Autodesk Inventor part; units mm, degrees
ref_plane "YZ Plane" through (0, 0, 0) normal (1, 0, 0) x (0, 1, 0)
ref_plane "XZ Plane" through (0, 0, 0) normal (0, 1, 0) x (-1, 0, 0)
ref_plane "XY Plane" through (0, 0, 0) normal (0, 0, 1) x (1, 0, 0)
sketch "Sketch1" plane through (0, 0, 0) normal (0, 0, 1) x (1, 0, 0)
  line L0 (0, 0) -> (9.5, 0)
  line L1 (9.5, 0) -> (9.5, 9.5)
  line L2 (9.5, 9.5) -> (0, 9.5)
  line L3 (0, 9.5) -> (0, 0)
  dimension "d0" = 9.5
  dimension "d1" = 9.5
extrude "Extrusion1" add sketch "Sketch1" along normal blind 9
sketch "Sketch2" plane through (9.5, 0, 0) normal (1, 0, 0) x (0, 0, -1)
  circle A0 centre (-15.25, 4.75) radius 4.75 construction
  line L0 (0, 0) -> (0, 9.5)
  line L1 (-9, 0) -> (-9, 9.5)
  line L2 (-9, 9.5) -> (-15.25, 9.5)
  line L3 (-9, 0) -> (-15.25, 0)
  arc A1 (-15.25, 9.5) -> (-15.25, 0) centre (-15.25, 4.75) ccw
  circle A2 centre (-15.25, 4.75) radius 1.5
  point P0 (0, 4.75)
  point P1 (0, 4.75)
  dimension "d4" = 9.5
  dimension "d5" = 15.25
  dimension "d6" = 3
extrude "Extrusion2" add sketch "Sketch2" against normal blind 3
sketch "Sketch3" plane through (0, 0, 0) normal (-1, 0, 0) x (0, 0, 1)
  circle A0 centre (15.25, 4.75) radius 1.5
  line L0 (9, 0) -> (9, 9.5)
  line L1 (9, 0) -> (15.25, 0)
  arc A1 (15.25, 0) -> (15.25, 9.5) centre (15.25, 4.75) ccw
  line L2 (15.25, 9.5) -> (9, 9.5)
  point P0 (0, 0)
extrude "Extrusion3" add sketch "Sketch3" against normal blind 3
fillet "Fillet1" radius 2 6 edges at (0, 4.75, 20) (0, 0, 7.625) (0, 9.5, 7.625) (9.5, 4.75, 20) (9.5, 0, 7.625) (9.5, 9.5, 7.625)
sketch "Sketch4" plane through (0, 0, 0) normal (0, 0, -1) x (-1, 0, 0)
  circle A0 centre (-4.75, 4.75) radius 2
  line L0 (-7.5, 9.5) -> (-2, 9.5)
  line L1 (0, 7.5) -> (0, 2)
  point P0 (0, 0)
  point P1 (0, 4.75)
  point P2 (-4.75, 9.5)
  dimension "d12" = 4
extrude "Extrusion4" cut sketch "Sketch4" against normal through all
sketch "Sketch5" plane through (0, 0, 9) normal (0, 0, 1) x (1, 0, 0)
  circle A0 centre (4.75, 4.75) radius 2
  circle A1 centre (4.75, 4.75) radius 3
  point P0 (0, 0)
  dimension "d15" = 6
extrude "Extrusion5" cut sketch "Sketch5" along normal blind 15 and the other way blind 6
properties part number "Arm6" material "ABS Plastic"
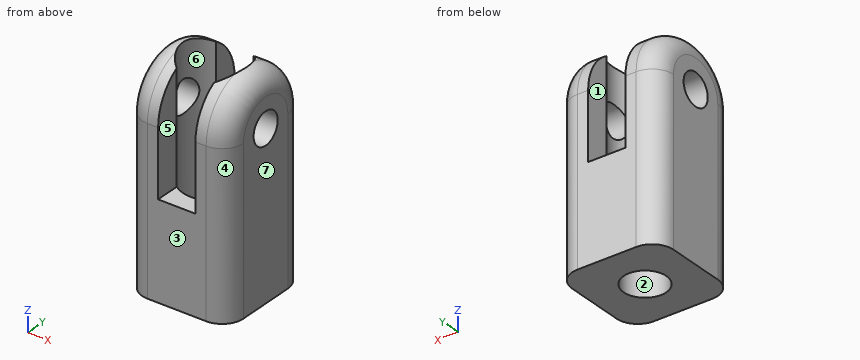
Here's how the part is built. I have some questions about the finished solid (model axes, mm). Face numbers are marked on the shaded views. A direction names the side the tool comes from. Round coordinates to 2 decimals unless told otherwise and drop trailing zeros. Write each loop counter-clockwise with the first axis right and the second up, starting at its lowest first coordinate (ties: lowest second). Pieces come first, ordered by that corner, then holes.
1. I need wall thicknesses on L1, parallel to X at y = 4.75, z = 13.25; L2, parallel to X at y = 2, z = 11; L3, parallel to Z at x = 6.25, y = 0.75. Which ranges of each line are inside material? Lowest first, please.
2. Suppose I cut it at C-C (z = 1.75). List the corners of the cut face in (x, y) for me, and give its area (4 significant figures).
3. If we mould it in two halves opening along X, with no side actions, what happens to the marked faces 1, 2, 3 and 4? For each: released by +X, released by -X, zero draft, split by the parting line, or undercut.
4. Suppose I cut it at B-B (x = 4.75). List the corners of the cut face in (y, z) for me, and give its area (3 significant figures).
5. For the marked faces 5, 6 and 7, which set-ups out of +Z, -Z, +X, -X, +Y, -Y let a thin tool reach every point of the face, with its end or its side?
6. Suppose I cut it at D-D (z = 11). List the corners of the cut face in (x, y) for me.
7. Suppose I cut it at A-A (y = 4.75). List the corners of the cut face in (x, z) for me.
8. Will these pins go through, and if not, where does the flat tip stop? pin 1 Ø1.2 at (x, y) = (4.5, 1) entering from +Z; pin 2 Ø1.2 at (y, z) = (0.5, 12.5) entering from +X; pin 3 Ø3 at (x, y) = (6, 4) entering from +Z.
Answer sheet:
1. L1: x = 0 to 1.75, 7.75 to 9.5
1. L2: x = 0 to 3, 6.5 to 9.5
1. L3: z = 0 to 9
2. outline: (0, 2) arc R2 ccw to (2, 0) - (7.5, 0) arc R2 ccw to (9.5, 2) - (9.5, 7.5) arc R2 ccw to (7.5, 9.5) - (2, 9.5) arc R2 ccw to (0, 7.5) - close; hole circle Ø4 at (4.75, 4.75)
2. area: 74.25 mm2
3. face 1: undercut
3. face 2: undercut
3. face 3: zero draft
3. face 4: released by +X
4. outline: (0, 0) - (2.75, 0) - (2.75, 3) - (1.75, 3) - (1.75, 9) - (0, 9) - close; (6.75, 0) - (9.5, 0) - (9.5, 9) - (7.75, 9) - (7.75, 3) - (6.75, 3) - close
4. area: 37.5 mm2
5. face 5: +Z, +Y, -Y
5. face 6: +Z
5. face 7: +Z, -Z, +X, +Y, -Y
6. outline: (0, 2) arc R2 ccw to (2, 0) - (3, 0) - (3, 2.31) arc R3 cw to (3, 7.19) - (3, 9.5) - (2, 9.5) arc R2 ccw to (0, 7.5) - close; (6.5, 0) - (7.5, 0) arc R2 ccw to (9.5, 2) - (9.5, 7.5) arc R2 ccw to (7.5, 9.5) - (6.5, 9.5) - (6.5, 7.19) arc R3 cw to (6.5, 2.31) - close
7. outline: (0, 0) - (2.75, 0) - (2.75, 3) - (1.75, 3) - (1.75, 13.75) - (0, 13.75) - close; (0, 16.75) - (1.75, 16.75) - (1.75, 19.98) arc R2 ccw to (0, 18) - close; (6.75, 0) - (9.5, 0) - (9.5, 13.75) - (7.75, 13.75) - (7.75, 3) - (6.75, 3) - close; (7.75, 16.75) - (9.5, 16.75) - (9.5, 18) arc R2 ccw to (7.75, 19.98) - close
8. pin 1: stops at z = 9
8. pin 2: stops at x = 9.29
8. pin 3: stops at z = 3
